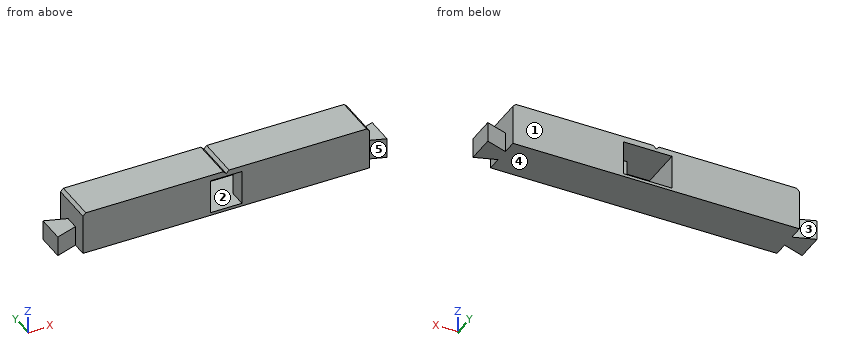
```python
from build123d import *

# Parameters (mm, degrees)
SKETCH1_W               = 100
SKETCH1_H               = 15
BODY_DEPTH              = 15
CLICK_DEPTH             = 7
CLICK_CHAMFER_SIZE      = 1
SKETCH4_W               = 2
SKETCH4_H               = 15
FIELDMARK_DEPTH         = 2
FIELDMARK_CHAMFER_SIZE  = 2
CUT_EXTRUDE1_DEPTH      = 62.241346327
CUT_EXTRUDE1_DEPTH_BACK = 62.241346327
SKETCH5_W               = 11
SKETCH5_H               = 12
SKETCH6_W               = 17
SKETCH6_H               = 12
CUT_EXTRUDE2_DEPTH      = 9


with BuildPart() as part:
    # Sketch1 → Body (new body)
    with BuildSketch(Plane.XY):
        Rectangle(SKETCH1_W, SKETCH1_H)
    extrude(amount=BODY_DEPTH)

    # Sketch2 → Click (add)
    with BuildSketch(Plane.XY):
        Polygon((-50, 0), (-50, 2.45), (-57.45, 4.95), (-57.45, 0), (-57.45, -4.95), (-50, -2.45), align=None)
        Polygon((57.45, 0), (57.45, -4.95), (50, -2.45), (50, 0), (50, 2.45), (57.45, 4.95), align=None)
    extrude(amount=CLICK_DEPTH)

    # Click Chamfer
    click_chamfer_edges = [part.edges().sort_by_distance(p)[0] for p in [
        (-50, 0, 15),
        (50, 0, 15),
    ]]
    chamfer(click_chamfer_edges, length=CLICK_CHAMFER_SIZE)

    # Sketch4 → FieldMark (cut)
    with BuildSketch(Plane.XY.offset(15)):
        Rectangle(SKETCH4_W, SKETCH4_H)
    extrude(amount=-FIELDMARK_DEPTH, mode=Mode.SUBTRACT)

    # FieldMark Chamfer
    # the kernel refuses this chamfer: 2 mm, written as the material it adds along each edge
    with BuildSketch(Plane(origin=(1, -7.5, 13), x_dir=(0.02749587661058638, 0, 0.9996219169112968), z_dir=(0, 1, 0))) as fieldmark_chamfer_piece_1_section:
        Polygon((FIELDMARK_CHAMFER_SIZE * 0.999621916911, -FIELDMARK_CHAMFER_SIZE * 0.0274958766106), (-FIELDMARK_CHAMFER_SIZE * 0.0274958766106, -FIELDMARK_CHAMFER_SIZE * 0.999621916911), (0, 0), align=None)
    fieldmark_chamfer_piece_1 = extrude(amount=15, mode=Mode.PRIVATE)
    fieldmark_chamfer_piece_1 = split(fieldmark_chamfer_piece_1, bisect_by=Plane(origin=(0.339191691, 0, 15), z_dir=(0, 0, -1)), keep=Keep.TOP, mode=Mode.PRIVATE)
    add(fieldmark_chamfer_piece_1)
    with BuildSketch(Plane(origin=(-1, 7.5, 13), x_dir=(0.9996219169112968, 0, -0.027495876610586487), z_dir=(0, -1, 0))) as fieldmark_chamfer_piece_2_section:
        Polygon((FIELDMARK_CHAMFER_SIZE * 0.999621916911, FIELDMARK_CHAMFER_SIZE * 0.0274958766106), (-FIELDMARK_CHAMFER_SIZE * 0.0274958766106, FIELDMARK_CHAMFER_SIZE * 0.999621916911), (0, 0), align=None)
    fieldmark_chamfer_piece_2 = extrude(amount=15, mode=Mode.PRIVATE)
    fieldmark_chamfer_piece_2 = split(fieldmark_chamfer_piece_2, bisect_by=Plane(origin=(-0.339191691, 0, 15), z_dir=(0, 0, -1)), keep=Keep.TOP, mode=Mode.PRIVATE)
    add(fieldmark_chamfer_piece_2)

    # Sketch5 → Cut-Extrude1 (cut, two sides: drawn at the far end of the back side and taken through both)
    with BuildSketch(Plane(origin=(0, 7.5, 0), x_dir=(1, 0, 0), z_dir=(0, 1, 0)).offset(-CUT_EXTRUDE1_DEPTH_BACK)):
        with Locations((0, -7)):
            Rectangle(SKETCH5_W, SKETCH5_H)
    extrude(amount=CUT_EXTRUDE1_DEPTH + CUT_EXTRUDE1_DEPTH_BACK, mode=Mode.SUBTRACT)

    # Sketch6 → Cut-Extrude2 (cut)
    with BuildSketch(Plane(origin=(0, 7.5, 0), x_dir=(1, 0, 0), z_dir=(0, 1, 0))):
        with Locations((3, -7)):
            Rectangle(SKETCH6_W, SKETCH6_H)
    extrude(amount=-CUT_EXTRUDE2_DEPTH, mode=Mode.SUBTRACT)


solid = part.part
```
Build history of the part. All positions in model axes, mm. Face numbers are marked on the shaded views. A direction names the side the tool comes from. Coordinates: 2 decimals unless noted, no trailing zeros. Order: outer loops, then holes, each group sorted by start corner. A loop starts at its lowest first (then second) coordinate and runs counter-clockwise, first axis right, second up. Notation, with made-up numbers: (40, 34) -> (46, 34) arc R11 cw to (46, 40) -> close; hole circle Ø6 at (67, -37). An arc over 180 degrees is marked (long way). Answer in a Markdown table with one row per item. Add a question column.
Q1. Band-saw the part on A-A, the plane x = 4. List the corners of the cut face in (y, z), then the cut area to 3 significant figures.
Q2. Band-saw the part on B-B, the plane z = 8.5. List the corners of the cut face in (x, y).
Q3. Wall check: line 1 along X through (y, z) = (1.75, 2); line 2 along X through (y, z) = (6, 4.25); line 3 along Z through (x, y) = (5, 7.25). Give the ranges that are in metal, low to high. Write a range as [from, to].
Q4. Drop flat-ended pins along their axis: pin 1 (3 mm diameter, centred on x = 9.5, z = 8, fed in from +Y); pin 2 (1.8 mm diameter, centred on y = -5, z = 6.5, fed in from -X); pin 3 (6 mm diameter, centred on x = 54, y = -0.5, fed in from +Z); pin 4 (5 mm diameter, centred on y = 4, z = 12.5, fed in from -X). Give the stop position or say it passes through.
Q5. Mould opens along X. For the marked faces 4 and 5 say: +X half, -X half, draft (parallel to the pull), parting line (faces both ways), or undercut.
Q6. Which spindle directions (+Z, -Z, +X, -X, +Y, -Y) get a long thin tool onto all of the face, cutting with end or side? Do the marked faces 1, 2 and 3. Say none if no direction does.
Answers follow:
| question | item | result |
|---|---|---|
| 1 | outline | (-7.5, 0) -> (7.5, 0) -> (7.5, 1) -> (-7.5, 1) -> close; (-7.5, 13) -> (7.5, 13) -> (7.5, 15) -> (-7.5, 15) -> close |
| 1 | area | 45.0 mm^2 |
| 2 | outline | (-50, -7.5) -> (-5.5, -7.5) -> (-5.5, 7.5) -> (-50, 7.5) -> close; (5.5, -7.5) -> (50, -7.5) -> (50, 7.5) -> (11.5, 7.5) -> (11.5, -1.5) -> (5.5, -1.5) -> close |
| 3 | line 1 | [-57.45, -5.5], [11.5, 57.45] |
| 3 | line 2 | [-50, -5.5], [11.5, 50] |
| 3 | line 3 | [0, 1], [13, 15] |
| 4 | pin 1 | y = -1.5 |
| 4 | pin 2 | x = -57.45 |
| 4 | pin 3 | z = 7 |
| 4 | pin 4 | x = -50 |
| 5 | face 4 | draft |
| 5 | face 5 | undercut |
| 6 | face 1 | +Z, -Z, +X, -X, +Y |
| 6 | face 2 | +Y |
| 6 | face 3 | +Z, -Z, +Y |
